Can you work these out from the model? Positions are in its coordinate system, mm. Round coordinates to 2 decimals unless told otherwise and drop trailing zeros. Order: outer loops, then holes, each group sorted by start corner. A loop starts at its lowest first (then second) coordinate and runs counter-clockwise, first axis right, second up.
Q1. Will these pins go through, and if not, where does the flat tip stop? P1, Ø3, axis at x = -420.5, y = -53.5, coming from the -Z side; P2, Ø6, axis at y = -55, z = -38.5, coming from the -X side; P3, Ø3, axis at y = -55.5, z = -62.5, coming from the +X side.
Q2. If I drill on line 1 (X direction, y = -56.5, z = -68.5); line 2 (Z direction, x = -413.25, y = -61.75) (3 decimals); line 3 (Y direction, x = -414.5, z = -33.5), over which ranges is the centre line in solid material (lowest first)?
Q3. If we section it at B-B (x = -421.25): Please give me the cut outline in (y, z) (3 decimals).
Q4. We'd pull the mould along X, two halves only. Please class faces 1 (the face through (-420.584, -59.873, 1.565)), 2 (the face through (-415, -51, 0)), 3 (the face through (-408.27, -52.63, 1.57)), 4 (the face through (-419.184, -56.042, -49.838)): pulls with the +X half, pulls with the -X half, needs draft (parallel to the pull), parting line crosses it, or undercut.
Q5. If we section it at A-A (z = -57.5): Please give me the cut outline in (x, y) (1 decimal).
Q6. If we section it at C-C (x = -407.25): Please give me the cut outline in (y, z) (3 decimals), plus the area to 3 significant figures.
Autodesk Inventor part; units mm, degrees
ref_plane "YZ Plane" through (0, 0, 0) normal (1, 0, 0) x (0, 1, 0)
ref_plane "XZ Plane" through (0, 0, 0) normal (0, 1, 0) x (-1, 0, 0)
ref_plane "XY Plane" through (0, 0, 0) normal (0, 0, 1) x (1, 0, 0)
sketch "Sketch1" plane through (0, 0, 0) normal (0, 0, 1) x (1, 0, 0)
  circle A0 centre (-414.4261, -56.251) radius 4.7625
  point P0 (0, 0)
  dimension "d0" = 9.525
extrude "Extrusion1" add sketch "Sketch1" against normal blind 101.6
sketch "Sketch2" plane through (-414.4261, -56.251, 0) normal (0, 0, 1) x (1, 0, 0)
  circle A0 centre (0, 0) radius 4.7625
  line L0 (-8.2489, 0) -> (-4.1244, 7.1437)
  line L1 (-4.1244, 7.1437) -> (4.1244, 7.1438)
  line L2 (4.1244, 7.1438) -> (8.2489, 0)
  line L3 (8.2489, 0) -> (4.1244, -7.1437)
  line L4 (4.1244, -7.1437) -> (-4.1244, -7.1438)
  line L5 (-4.1244, -7.1438) -> (-8.2489, 0)
  point P0 (414.4261, 56.251)
  dimension "d3" = 14.2875
extrude "Extrusion2" add sketch "Sketch2" along normal blind 3.175 contours A0 | L0 L1 L2 L3 L4 L5
thread "Thread1"
chamfer "Chamfer1" distance 0.508 angle 45 1 edges at (-419.1886, -56.251, -101.6)
properties part number "375 bolt x4" material "Steel"
Solution:
1. P1: stops at z = 0
1. P2: stops at x = -419.19
1. P3: stops at x = -409.66
2. line 1: x = -419.18 to -409.67
2. line 2: z = 0 to 3.175
2. line 3: y = -61.01 to -51.49
3. outline: (-58.719, 0) - (-53.783, 0) - (-53.783, 3.175) - (-58.719, 3.175) - close
4. face 1: pulls with the -X half
4. face 2: needs draft
4. face 3: pulls with the +X half
4. face 4: parting line crosses it
5. outline: circle Ø9.5 at (-414.4, -56.3)
6. outline: (-58.109, 0) - (-54.393, 0) - (-54.393, 3.175) - (-58.109, 3.175) - close
6. area: 11.8 mm2
